Autodesk Fusion 360 part; units mm, degrees
sketch "Sketch1" plane through (0, 0, 0) normal (0, 0, 1) x (1, 0, 0)
  circle A0 centre (0, 0) radius 9
  line L0 (0, 9) -> (25, 9)
  line L1 (25, 9) -> (25, 3)
  line L2 (25, 3) -> (19, 3)
  arc A1 (19, 3) -> (7.8189, -4.457) centre (20.8503, -11.8854) ccw
  dimension "d1" = 18
  dimension "d2" = 25
  dimension "d3" = 6
  dimension "d4" = 6
  dimension "d5" = 15
extrude "Extrude1" add sketch "Sketch1" along normal mid plane 20
shell "Shell1" thickness 1 removed faces 1 at (25, 7, 3.3333)
sketch "Sketch2" plane through (0, 0, 0) normal (0, 0, 1) x (1, 0, 0)
  line L0 (0, 9) -> (25, 9)
  line L1 (0, 8) -> (25, 8)
  line L2 (2, 9) -> (3, 8)
  line L3 (2, 9) -> (1.4972, 9) construction
  line L4 (7, 9) -> (6, 8)
  line L5 (7, 9) -> (6.4972, 9) construction
  dimension "d9" = 45
  dimension "d10" = 135
  dimension "d11" = 3
  dimension "d12" = 2
extrude "Extrude2" cut sketch "Sketch2" along normal mid plane 15
sketch "Sketch3" plane through (0, 0, 0) normal (0, 0, 1) x (1, 0, 0)
  line L0 (-11.6458, 2.5) -> (-8.6458, 2.5)
  line L1 (-8.6458, 2.5) -> (-8.6458, -2.5)
  line L2 (-8.6458, -2.5) -> (-11.6458, -2.5)
  line L3 (-11.6458, -2.5) -> (-11.6458, 2.5)
  arc A0 (0, 9) -> (7.8189, -4.457) centre (0, 0) ccw
  arc A1 (-11.6458, 2.5) -> (-11.6458, -2.5) centre (-11.6458, 0) ccw
  circle A2 centre (-11.6458, 0) radius 1.5
  dimension "d15" = 3
  dimension "d16" = 5
  dimension "d17" = 3
extrude "Extrude3" add sketch "Sketch3" along normal mid plane 3 contours L0 L2 L3 A0 A2 | L3 A1 A2
fillet "Fillet1" radius 0.5 18 edges at (12.5, 9, 10) (-7.7818, -4.5214, 10) (12.5275, 0.5938, 10) (25, 9, 0) (25, 6, 10) (22, 3, 10) (25, 3, 0) (25, 6, -10) (12.5275, 0.5938, -10) (-7.7818, -4.5214, -10) (12.5, 9, -10) (22, 3, -10) (-10.1458, 2.5, 1.5) (-14.1458, 0, 1.5) (-10.1458, -2.5, 1.5) (-10.1458, -2.5, -1.5) (-14.1458, 0, -1.5) (-10.1458, 2.5, -1.5)
chamfer "Chamfer1" distance 0.5 angle 45 4 edges at (25, 4, 0) (25, 6, -9) (25, 8, 0) (25, 6, 9)
Read the model definition and answer for the solid it produces. Units are mm, in the model's axes. A direction names the side the tool comes from. Round coordinates to 2 decimals unless told otherwise and drop trailing zeros.
1) The mould has two halves that part along Y. Classify faces 1 (the face through (22, 3, 0)), 2 (the face through (-10, 1, -1.5)), 3 (the face through (11.912, 1.385, -0.126)), 4 (the face through (-13.144, -0.066, -0.021)): released by +Y, released by -Y, zero draft, split by the parting line, or undercut.
2) Flat-ended cylindrical pins translate along their axes: pin 1 (12 mm diameter, centred on x = 10, z = 1, fed in from -Y); pin 2 (1 mm diameter, centred on x = -10, z = 0.5, fed in from -Y); pin 3 (8 mm diameter, centred on y = -0.5, z = 7.5, fed in from -X). Find the tip coordinate at first contact, or state that the pin passes through.
3) For faces 5 (the face through (-10, 2.5, 0)), 6 (the face through (4.5, 8.5, -7.5)), 7 (the face through (4, 2, 9)), 8 (the face through (-10, -2.5, 0)), 9 (the face through (22, 4, 0)), determine the directions among +Z, -Z, +X, -X, +Y, -Y from which every point of the face is accessible in a straight line to the end or side of a thin tool.
4) The part is cut by section C-C on y = 0. Give the number of separate pieces and of enclosed holes in the cut face, plus the area to 3 significant figures.
5) Straight lines are drawn through the part: L1, parallel to Z at x = 12, y = 1.5; L2, parallel to Y at x = 22.5, z = -8.75; L3, parallel to Y at x = 0, z = 3.25. For each, find the intervals that lie inside material, in ascending order.
Resolved:
1. face 1: released by -Y
1. face 2: zero draft
1. face 3: undercut
1. face 4: undercut
2. pin 1: stops at y = -8.06
2. pin 2: stops at y = -2.5
2. pin 3: stops at x = -9
3. face 5: +Z, -Z, -X, +Y
3. face 6: +Y
3. face 7: none
3. face 8: +Z, -Z, -X, -Y
3. face 9: +X
4. separate pieces: 2
4. enclosed holes: 1
4. area: 93.5 mm2
5. L1: z = -10 to -9, 9 to 10
5. L2: y = 3 to 4, 8 to 9
5. L3: y = -9 to -8, 8 to 9
